CAD build for the part. Positions are in the model's coordinates, mm. Round coordinates to 2 decimals unless told otherwise and drop trailing zeros. Write each loop counter-clockwise with the first axis right and the second up, starting at its lowest first coordinate (ties: lowest second). Pieces come first, ordered by that corner, then holes. Notation, with made-up numbers: (39.25, 37) - (61.25, 37) arc R13 ccw to (61.25, 53) - close; hole circle Ø6 at (-10, -39). An arc over 180 degrees is marked (long way). Use one line per item in the form item = value. Start each with the question number.
Item 1: Drill centre lines: L1, parallel to Y at x = -5, z = 0.6; L2, parallel to Y at x = -25, z = 0.75; L3, parallel to Y at x = -26, z = 0.8. Where is each one in solid material? Low to high.
Item 2: Band-saw the part on C-C, the plane z = 0.7. List the corners of the cut face in (x, y), and give its area (3 significant figures).
Item 3: Band-saw the part on B-B, the plane y = 7. List the corners of the cut face in (x, z).
Item 4: Band-saw the part on A-A, the plane x = -5. List the corners of the cut face in (y, z), and give its area (3 significant figures).
Item 5: Band-saw the part on D-D, the plane y = 25. List the corners of the cut face in (x, z), and give its area (3 significant figures).
Item 6: Pull direction X, two halves, no side cores. Call faces 1 (the cylindrical face through (-1.204, 35.006, 1.014)), 2 (the cylindrical face through (-26.84, 6.69, 1.01)), 3 (the flat face through (-14, 14, 2)), 4 (the cylindrical face through (-3.66, 27.11, 1.01)): +X half, -X half, draft (parallel to the pull), parting line (faces both ways), or undercut.
from build123d import *

# Parameters (mm, degrees)
BOSS_EXTRUDE1_DEPTH   = 2
F_5_0MM_DOWEL_HOLE1_D = 5
FILLET1_R             = 2


with BuildPart() as part:
    # Sketch1 → Boss-Extrude1 (new body)
    with BuildSketch(Plane.XY):
        Polygon((0, 0), (0, 38), (-38, 0), align=None)
    extrude(amount=BOSS_EXTRUDE1_DEPTH)

    # Ø5.0mm Dowel Hole1 (through all)
    with Locations(Plane(origin=(0, 0, 0), x_dir=(-1, 0, 0), z_dir=(0, 0, -1))):
        with Locations((5, 25), (5, 5), (25, 5)):
            Hole(F_5_0MM_DOWEL_HOLE1_D / 2)

    # Fillet1
    fillet1_edges = [part.edges().sort_by_distance(p)[0] for p in [
        (-38, 0, 1),
        (0, 38, 1),
        (0, 0, 1),
    ]]
    fillet(fillet1_edges, radius=FILLET1_R)


solid = part.part
Determined:
q1.L1 = 0 to 2.5, 7.5 to 22.5, 27.5 to 33
q1.L2 = 0 to 2.5, 7.5 to 13
q1.L3 = 0 to 2.71, 7.29 to 12
q2.outline = (-34.59, 3.41) arc R2 ccw to (-33.17, 0) - (-2, 0) arc R2 ccw to (0, 2) - (0, 33.17) arc R2 ccw to (-3.41, 34.59) - close; hole circle Ø5 at (-25, 5); hole circle Ø5 at (-5, 5); hole circle Ø5 at (-5, 25)
q2.area = 652 mm²
q3.outline = (-31, 0) - (-26.5, 0) - (-26.5, 2) - (-31, 2) - close; (-23.5, 0) - (-6.5, 0) - (-6.5, 2) - (-23.5, 2) - close; (-3.5, 0) - (0, 0) - (0, 2) - (-3.5, 2) - close
q4.outline = (0, 0) - (2.5, 0) - (2.5, 2) - (0, 2) - close; (7.5, 0) - (22.5, 0) - (22.5, 2) - (7.5, 2) - close; (27.5, 0) - (33, 0) - (33, 2) - (27.5, 2) - close
q4.area = 46.0 mm²
q5.outline = (-13, 0) - (-7.5, 0) - (-7.5, 2) - (-13, 2) - close; (-2.5, 0) - (0, 0) - (0, 2) - (-2.5, 2) - close
q5.area = 16.0 mm²
q6.face_1 = parting line
q6.face_2 = undercut
q6.face_3 = draft
q6.face_4 = undercut
